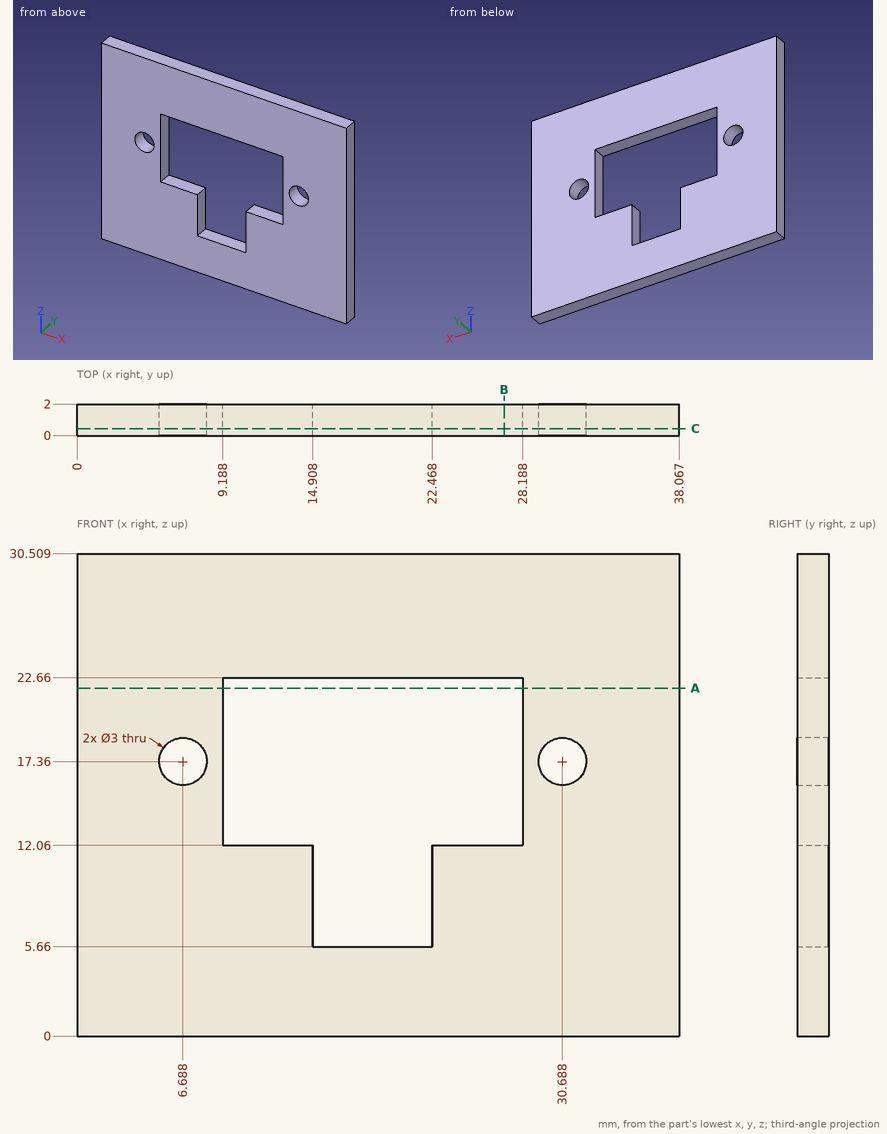
The figure shows three views and two pictorial views of one solid part (mm, origin at its lowest corner). Answer the questions. Round coordinates to 2 decimals unless told otherwise and drop trailing zeros. Write each loop counter-clockwise with the first axis right and the second up, starting at its lowest first coordinate (ties: lowest second). Pieces come first, ordered by that corner, then holes. Notation, with made-up numbers: (-0.75, 81) - (31.25, 81) arc R10 ccw to (31.25, 86) - close; hole circle Ø2 at (67.5, -19.5). An arc over 180 degrees is marked (long way). One line per question, with ' | ' between items. Start each with the question number.
1. Section A-A (z = 22) is taken. Determine the outline of the cut face in (x, y).
2. Section C-C (y = 0.45) is taken. Determine the outline of the cut face in (x, z).
3. Section B-B (x = 27) is taken. Determine the outline of the cut face in (y, z).
4. This flat-tipped pin is pushed along its axis until it touches: pin 1 (0.6 mm diameter, centred on y = 0.5, z = 17, fed in from -X). Where does it stop, or does it pass through?
5. Find the intervals of material crossed by probe 1 along X at (y, z) = (1.75, 11.5); probe 2 along Z at (x, y) = (16, 0.4); probe 3 along X at (y, z) = (1.8, 13), in increasing order. Write a range as [from, to].
Filled in:
1) outline: (0, 0) - (9.19, 0) - (9.19, 2) - (0, 2) - close; (28.19, 0) - (38.07, 0) - (38.07, 2) - (28.19, 2) - close
2) outline: (0, 0) - (38.07, 0) - (38.07, 30.51) - (0, 30.51) - close; hole circle Ø3 at (6.69, 17.36); hole (9.19, 12.06) - (14.91, 12.06) - (14.91, 5.66) - (22.47, 5.66) - (22.47, 12.06) - (28.19, 12.06) - (28.19, 22.66) - (9.19, 22.66) - close; hole circle Ø3 at (30.69, 17.36)
3) outline: (0, 0) - (2, 0) - (2, 12.06) - (0, 12.06) - close; (0, 22.66) - (2, 22.66) - (2, 30.51) - (0, 30.51) - close
4) pin 1: x = 0
5) probe 1: [0, 14.91], [22.47, 38.07] | probe 2: [0, 5.66], [22.66, 30.51] | probe 3: [0, 9.19], [28.19, 38.07]
